from build123d import *

# Parameters (mm, degrees)
SKICA1_R                = 1.25
SKICA1_R_2              = 1.5
P_IDAT_VYSUNUT_M1_DEPTH = 0.5


with BuildPart() as part:
    # Skica1 → Přidat vysunutím1 (new, symmetric)
    with BuildSketch(Plane(origin=(0, 0, 0), x_dir=(1, 0, 0), z_dir=(0, 1, 0))):
        with BuildLine():
            Line((-29.963432056, -9.556318536), (-22.961281, -62.589043156))
            ThreePointArc((-22.961281, -62.589043156), (-21.466420891, -65.383836152), (-18.5, -66.5))
            Line((-18.5, -66.5), (18.5, -66.5))
            ThreePointArc((18.5, -66.5), (21.466420891, -65.383836152), (22.961281, -62.589043156))
            Line((22.961281, -62.589043156), (29.963432056, -9.556318536))
            ThreePointArc((29.963432056, -9.556318536), (29.99084816, -9.278759542), (30, -9))
            Line((30, -9), (30, 9))
            ThreePointArc((30, 9), (27.693135825, 12.77977819), (23.276836158, 12.4562929))
            ThreePointArc((23.276836158, 12.4562929), (0, 4.986108431), (-23.276836158, 12.4562929))
            ThreePointArc((-23.276836158, 12.4562929), (-27.693135825, 12.77977819), (-30, 9))
            Line((-30, 9), (-30, -9))
            ThreePointArc((-30, -9), (-29.99084816, -9.278759542), (-29.963432056, -9.556318536))
        make_face()
        with Locations(Location((-25.75, 9, 0), (0, 0, 270))):
            Circle(SKICA1_R, mode=Mode.SUBTRACT)
        with Locations(Location((25.75, 9, 0), (0, 0, 270))):
            Circle(SKICA1_R, mode=Mode.SUBTRACT)
        with Locations(Location((-25.75, -9, 0), (0, 0, 270))):
            Circle(SKICA1_R, mode=Mode.SUBTRACT)
        with Locations(Location((25.75, -9, 0), (0, 0, 270))):
            Circle(SKICA1_R, mode=Mode.SUBTRACT)
        with Locations(Location((-18.5, -62, 0), (0, 0, 270))):
            Circle(SKICA1_R_2, mode=Mode.SUBTRACT)
        with Locations(Location((18.5, -62, 0), (0, 0, 270))):
            Circle(SKICA1_R_2, mode=Mode.SUBTRACT)
    extrude(amount=P_IDAT_VYSUNUT_M1_DEPTH, both=True)


solid = part.part
For this review, take the finished solid that the model builds, in its own axes (mm). Round coordinates to 2 decimals unless told otherwise and drop trailing zeros. Loops run counter-clockwise (first coordinate to the right, second up) from the corner with the lowest first, then second, coordinate; pieces in that order, holes last. Notation, with made-up numbers: (56, 24) - (88, 24) arc R15 ccw to (88, 41) - close; hole circle Ø4 at (74, 3). An arc over 180 degrees is marked (long way). One line per item, written item: value. Start each with the question number.
Item 1: The part is to be moulded in two halves that separate along Z. For faces 1 (the cylindrical face through (27.75, 0.01, -12.75)), 2 (the cylindrical face through (25.8, -0.01, -10.25)), 3 (the flat face through (26.413, 0.007, 36.444)), say which applies: +Z half, -Z half, draft (parallel to the pull), parting line (faces both ways), or undercut.
Item 2: Take a section at D-D (x = 5). Give the boundary of the cut face in (y, z).
Item 3: For L1, parallel to X at y = 0.25, z = 9; L2, parallel to X at y = 0.05, z = -9; L3, parallel to X at y = 0.15, z = 62, list the stretches that pass through material, from the lowest coordinate up.
Item 4: Take a section at A-A (y = 0.2). Give the boundary of the cut face in (x, z).
Item 5: Take a section at B-B (x = 25.75). Give the boundary of the cut face in (y, z).
Item 6: Take a section at C-C (z = 42.5). Give the boundary of the cut face in (x, y), plus the area to 3 significant figures.
Answer below:
1. face 1: -Z half
1. face 2: undercut
1. face 3: +Z half
2. outline: (-0.5, -5.3) - (0.5, -5.3) - (0.5, 66.5) - (-0.5, 66.5) - close
3. L1: x = -30 to -27, -24.5 to 24.5, 27 to 30
3. L2: x = -30 to -27, -24.5 to -17.46, 17.46 to 24.5, 27 to 30
3. L3: x = -23.04 to -20, -17 to 17, 20 to 23.04
4. outline: (-30, -9) arc R4.25 ccw to (-23.28, -12.46) arc R40 cw to (23.28, -12.46) arc R4.25 ccw to (30, -9) - (30, 9) arc R4.25 ccw to (29.96, 9.56) - (22.96, 62.59) arc R4.5 ccw to (18.5, 66.5) - (-18.5, 66.5) arc R4.5 ccw to (-22.96, 62.59) - (-29.96, 9.56) arc R4.25 ccw to (-30, 9) - close; hole circle Ø2.5 at (-25.75, -9); hole circle Ø2.5 at (-25.75, 9); hole circle Ø3 at (-18.5, 62); hole circle Ø3 at (18.5, 62); hole circle Ø2.5 at (25.75, -9); hole circle Ø2.5 at (25.75, 9)
5. outline: (-0.5, -13.25) - (0.5, -13.25) - (0.5, -10.25) - (-0.5, -10.25) - close; (-0.5, -7.75) - (0.5, -7.75) - (0.5, 7.75) - (-0.5, 7.75) - close; (-0.5, 10.25) - (0.5, 10.25) - (0.5, 41.47) - (-0.5, 41.47) - close
6. outline: (-25.61, -0.5) - (25.61, -0.5) - (25.61, 0.5) - (-25.61, 0.5) - close
6. area: 51.2 mm2
